For this review, take the finished solid that the model builds, in its own axes (mm). Coordinates: 2 decimals unless noted, no trailing zeros. Write each loop counter-clockwise with the first axis right and the second up, starting at its lowest first coordinate (ties: lowest second). Pieces come first, ordered by that corner, then holes.
1) Insertion check: P1, Ø1.5, axis at x = -1, z = 2, coming from the -Y side; P2, Ø1.5, axis at y = 40, z = 1, coming from the +X side; P3, Ø3.5, axis at x = -5, y = -56.25, coming from the -Z side; P4, Ø1.2, axis at x = -8, z = 1.5, coming from the +Y side. Each pin has a flat end and moves straight along its axis. Give the tip position at first contact, or say it passes through.
2) We need section B-B on z = 1.05. Give the number of separate pieces and of enclosed holes in the cut face, then the cut area to 3 significant figures.
3) We need section A-A on x = -5. Write out the cut boundary in (y, z).
4) To check wall thickness, follow line 1 along Y through (x, z) = (-5, 0.95); line 2 along Y through (x, z) = (-0.75, 3.35); line 3 along Y through (x, z) = (-3.75, 0.55). State the ranges of each line that lie inside material, in increasing order.
from build123d import *

# Parameters (mm, degrees)
CROQUIS1_W              = 10
CROQUIS1_H              = 4
CROQUIS1_R              = 2
SALIENTE_EXTRUIR1_DEPTH = 4


with BuildPart() as part:
    # Croquis1 → Saliente-Extruir1 (new body)
    with BuildSketch(Plane.XY):
        with BuildLine():
            Line((-14, -70), (-10, -70))
            Line((-10, -70), (-10, -66))
            Line((-10, -66), (-7, -66))
            Line((-7, -66), (-7, -64.5))
            Line((-7, -64.5), (-9.5, -64.5))
            Line((-9.5, -64.5), (-9.5, -61.5))
            Line((-9.5, -61.5), (-0.5, -61.5))
            Line((-0.5, -61.5), (-0.5, -64.5))
            Line((-0.5, -64.5), (-3, -64.5))
            Line((-3, -64.5), (-3, -66))
            Line((-3, -66), (0, -66))
            Line((0, -66), (0, -70))
            Line((0, -70), (4, -70))
            ThreePointArc((4, -70), (4.707106781, -69.707106781), (5, -69))
            Line((5, -69), (5, -66.298618771))
            ThreePointArc((5, -66.298618771), (4.959256868, -66.016083354), (4.840347477, -65.756570693))
            add(Edge.make_bspline(
                [(4.840347477, -65.756570693), (3.280115826, -63.337713796), (1.719884174, -58.5), (3.280115826, -53.662286204), (4.840347477, -51.243429307)],
                knots=[0.01622862, 0.01622862, 0.01622862, 0.01622862, 0.5, 0.98377138, 0.98377138, 0.98377138, 0.98377138], degree=3))
            ThreePointArc((4.840347477, -51.243429307), (4.959256868, -50.983916646), (5, -50.701381229))
            Line((5, -50.701381229), (5, -47.070997241))
            ThreePointArc((5, -47.070997241), (4.997494145, -47.000248166), (4.989989137, -46.929853666))
            add(Edge.make_bspline(
                [(4.989989137, -46.929853666), (3.329996379, -35.286569111), (1.670003621, -12), (3.329996379, 11.286569111), (4.989989137, 22.929853666)],
                knots=[0.00100209, 0.00100209, 0.00100209, 0.00100209, 0.5, 0.99899791, 0.99899791, 0.99899791, 0.99899791], degree=3))
            ThreePointArc((4.989989137, 22.929853666), (4.997494145, 23.000248166), (5, 23.070997241))
            Line((5, 23.070997241), (5, 26.838505544))
            ThreePointArc((5, 26.838505544), (4.987329796, 26.997187218), (4.949640253, 27.151847833))
            add(Edge.make_bspline(
                [(4.949640253, 27.151847833), (1.666752066, 37.101231889), (1.683538525, 47.056062614), (5, 57)],
                knots=[0.005061594, 0.005061594, 0.005061594, 0.005061594, 1, 1, 1, 1], degree=3))
            Line((5, 57), (5, 69))
            ThreePointArc((5, 69), (4.707106781, 69.707106781), (4, 70))
            Line((4, 70), (0, 70))
            Line((0, 70), (0, 66))
            Line((0, 66), (-3, 66))
            Line((-3, 66), (-3, 61))
            Line((-3, 61), (0, 61))
            Line((0, 61), (0, 57))
            Line((0, 57), (-10, 57))
            Line((-10, 57), (-10, 61))
            Line((-10, 61), (-7, 61))
            Line((-7, 61), (-7, 66))
            Line((-7, 66), (-10, 66))
            Line((-10, 66), (-10, 70))
            Line((-10, 70), (-14, 70))
            ThreePointArc((-14, 70), (-14.707106781, 69.707106781), (-15, 69))
            Line((-15, 69), (-15, 57))
            add(Edge.make_bspline(
                [(-14.949640253, 27.151847833), (-11.666752066, 37.101231889), (-11.683538525, 47.056062614), (-15, 57)],
                knots=[0.005061594, 0.005061594, 0.005061594, 0.005061594, 1, 1, 1, 1], degree=3))
            ThreePointArc((-14.949640253, 27.151847833), (-14.987329796, 26.997187218), (-15, 26.838505544))
            Line((-15, 26.838505544), (-15, 23.070997241))
            ThreePointArc((-15, 23.070997241), (-14.997494145, 23.000248166), (-14.989989137, 22.929853666))
            add(Edge.make_bspline(
                [(-14.989989137, -46.929853666), (-13.329996379, -35.286569111), (-11.670003621, -12), (-13.329996379, 11.286569111), (-14.989989137, 22.929853666)],
                knots=[0.00100209, 0.00100209, 0.00100209, 0.00100209, 0.5, 0.99899791, 0.99899791, 0.99899791, 0.99899791], degree=3))
            ThreePointArc((-14.989989137, -46.929853666), (-14.997494145, -47.000248166), (-15, -47.070997241))
            Line((-15, -47.070997241), (-15, -50.701381229))
            ThreePointArc((-15, -50.701381229), (-14.959256868, -50.983916646), (-14.840347477, -51.243429307))
            add(Edge.make_bspline(
                [(-14.840347477, -51.243429307), (-13.280115826, -53.662286204), (-11.719884174, -58.5), (-13.280115826, -63.337713796), (-14.840347477, -65.756570693)],
                knots=[0.01622862, 0.01622862, 0.01622862, 0.01622862, 0.5, 0.98377138, 0.98377138, 0.98377138, 0.98377138], degree=3))
            ThreePointArc((-14.840347477, -65.756570693), (-14.959256868, -66.016083354), (-15, -66.298618771))
            Line((-15, -66.298618771), (-15, -69))
            ThreePointArc((-15, -69), (-14.707106781, -69.707106781), (-14, -70))
        make_face()
        with Locations((-5, 25)):
            Rectangle(CROQUIS1_W, CROQUIS1_H, mode=Mode.SUBTRACT)
        with Locations((-5, -49)):
            Rectangle(CROQUIS1_W, CROQUIS1_H, mode=Mode.SUBTRACT)
        with Locations((-5, -56.25)):
            Circle(CROQUIS1_R, mode=Mode.SUBTRACT)
    extrude(amount=SALIENTE_EXTRUIR1_DEPTH)


solid = part.part
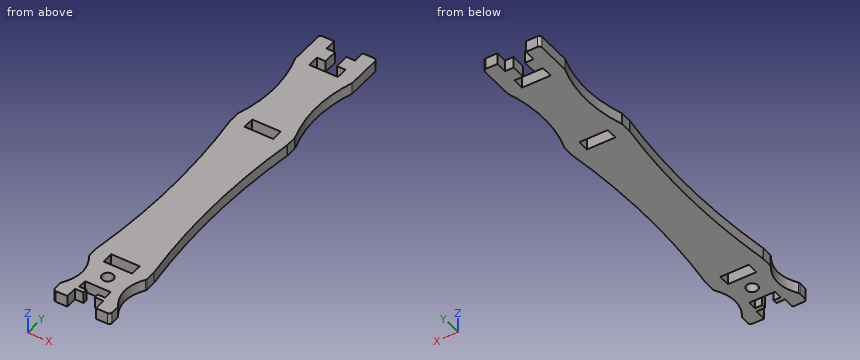
Result:
1. P1: stops at y = -66
1. P2: stops at x = 2.58
1. P3: passes through
1. P4: stops at y = 66
2. separate pieces: 1
2. enclosed holes: 3
2. area: 2,150 mm2
3. outline: (-61.5, 0) - (-58.25, 0) - (-58.25, 4) - (-61.5, 4) - close; (-54.25, 0) - (-51, 0) - (-51, 4) - (-54.25, 4) - close; (-47, 0) - (23, 0) - (23, 4) - (-47, 4) - close; (27, 0) - (57, 0) - (57, 4) - (27, 4) - close
4. line 1: y = -61.5 to -58.25, -54.25 to -51, -47 to 23, 27 to 57
4. line 2: y = -66 to -64.5, -61.5 to -51, -47 to 23, 27 to 57, 61 to 66
4. line 3: y = -61.5 to -57.81, -54.69 to -51, -47 to 23, 27 to 57
